Design review of the part built by this model. Coordinates are the model's own, in mm. Face numbers are marked on the shaded views. A direction names the side the tool comes from. Coordinates: 2 decimals unless noted, no trailing zeros. Order: outer loops, then holes, each group sorted by start corner. A loop starts at its lowest first (then second) coordinate and runs counter-clockwise, first axis right, second up. Notation, with made-up numbers: (31.25, 73) - (76.25, 73) arc R33 cw to (76.25, 108) - close; hole circle Ø6 at (-34.75, 49). An arc over 180 degrees is marked (long way). Write each question's results on one line, items separated by ' | '. Start each with the question number.
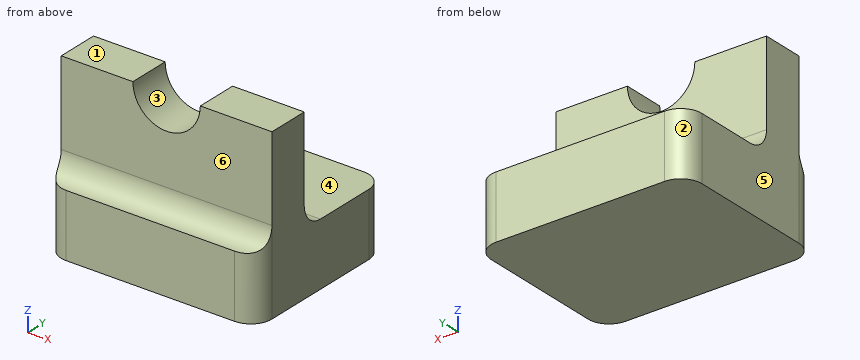
```python
from build123d import *

# Parameters (mm, degrees)
F0_W        = 50
F0_H        = 40
F1_DEPTH    = 15
F2_W        = 50
F2_H        = 10
F3_DEPTH    = 25
F5_DEPTH    = 25
F7_T1_DEPTH = 50
F7_T3_DEPTH = 40


# Not quite as in the source:
# - a fillet or chamfer that OpenCascade refuses, or shapes differently, is made with other operations: its cross-section is extruded or revolved along the edge and cut away or added
# - a feature of the source that left no trace in its solid (it failed there, or was rolled back) is left out


with BuildPart() as f1:
    # F0 (on Top) → F1 (new body)
    with BuildSketch(Plane.XY):
        with Locations((29.4554777443, -26.2415218353)):
            Rectangle(F0_W, F0_H)
    extrude(amount=F1_DEPTH)

    # F2 (on face) → F3 (join)
    with BuildSketch(Plane.XY.offset(15)):
        with Locations((29.4554777443, -36.2415218353)):
            Rectangle(F2_W, F2_H)
    extrude(amount=F3_DEPTH)

    # F4 (on face) → F5 (cut)
    with BuildSketch(Plane(origin=(0, -31.2415218353, 0), x_dir=(-1, 0, 0), z_dir=(0, 1, 0))):
        with BuildLine():
            ThreePointArc((-37.4554777443, 40), (-29.4554777443, 32), (-21.4554777443, 40))
            Line((-21.4554777443, 40), (-37.4554777443, 40))
        make_face()
    extrude(amount=-F5_DEPTH, mode=Mode.SUBTRACT)

    # F7: fillet of radius 5 on 6 edges, made by hand

    # F7_s2 → F7_t1 (join)
    with BuildSketch(Plane.YZ.offset(4.4554777443)):
        with BuildLine():
            ThreePointArc((-46.2415218353, 15), (-42.7059879294, 16.4644660941), (-41.2415218353, 20))
            Line((-41.2415218353, 20), (-41.2415218353, 15))
            Line((-41.2415218353, 15), (-46.2415218353, 15))
        make_face()
        with BuildLine():
            ThreePointArc((-26.2415218353, 15), (-29.7770557413, 16.4644660941), (-31.2415218353, 20))
            Line((-31.2415218353, 20), (-31.2415218353, 15))
            Line((-31.2415218353, 15), (-26.2415218353, 15))
        make_face()
    extrude(amount=F7_T1_DEPTH)

    # F7_s4 → F7_t3 (cut)
    with BuildSketch(Plane.XY.offset(-12.5)):
        with BuildLine():
            ThreePointArc((9.4554777443, -46.2415218353), (5.9199438384, -44.7770557413), (4.4554777443, -41.2415218353))
            Line((4.4554777443, -41.2415218353), (4.4554777443, -46.2415218353))
            Line((4.4554777443, -46.2415218353), (9.4554777443, -46.2415218353))
        make_face()
        with BuildLine():
            ThreePointArc((49.4554777443, -46.2415218353), (52.9910116503, -44.7770557413), (54.4554777443, -41.2415218353))
            Line((54.4554777443, -41.2415218353), (54.4554777443, -46.2415218353))
            Line((54.4554777443, -46.2415218353), (49.4554777443, -46.2415218353))
        make_face()
        with BuildLine():
            ThreePointArc((4.4554777443, -11.2415218353), (5.9199438384, -7.7059879294), (9.4554777443, -6.2415218353))
            Line((9.4554777443, -6.2415218353), (4.4554777443, -6.2415218353))
            Line((4.4554777443, -6.2415218353), (4.4554777443, -11.2415218353))
        make_face()
        with BuildLine():
            ThreePointArc((54.4554777443, -11.2415218353), (52.9910116503, -7.7059879294), (49.4554777443, -6.2415218353))
            Line((49.4554777443, -6.2415218353), (54.4554777443, -6.2415218353))
            Line((54.4554777443, -6.2415218353), (54.4554777443, -11.2415218353))
        make_face()
    extrude(amount=F7_T3_DEPTH, mode=Mode.SUBTRACT)


solid = f1.part
```
(1) Mouldability with a two-part tool opening along X and no side actions: class the marked faces 1, 2 and 3 as +X half, -X half, draft (parallel to the pull), parting line (faces both ways), or undercut.
(2) To check wall thickness, follow line 1 along Y through (x, z) = (20.5, 32.5); line 2 along Z through (x, y) = (33, -12.5); line 3 along Z through (x, y) = (13.5, -27.5). State the ranges of each line that lie inside material, in increasing order. Write a range as [from, to].
(3) Take a section at D-D (z = 22). State the section outline as (x, y) points, plus the area to 3 significant figures.
(4) Clearance check with flat-ended pins moving along their axes: pin 1 (6 mm diameter, centred on x = 28.5, y = -12, fed in from -Z); pin 2 (5 mm diameter, centred on x = 42, z = 32.5, fed in from -Y); pin 3 (22 mm diameter, centred on x = 21, y = -16.5, fed in from +Z); pin 4 (6 mm diameter, centred on x = 31, z = 27.5, fed in from +Y). State where each tip first meets the part, or that it passes through.
(5) Tool access review of the marked faces 4, 5 and 6: name each direction out of +Z, -Z, +X, -X, +Y, -Y from which nothing blocks a thin tool from reaching the whole face with its end or side.
(6) Take a section at A-A (x = 39). State the section outline as (y, z) points, plus the area to 3 significant figures.
(7) Take a section at C-C (y = -38). State the section outline as (x, z) points.
(8) Take a section at B-B (z = 36). State the section outline as (x, y) points.
Worked out:
1) face 1: draft | face 2: -X half | face 3: undercut
2) line 1: [-41.24, -31.24] | line 2: [0, 15] | line 3: [0, 15.16]
3) outline: (4.46, -41.24) - (54.46, -41.24) - (54.46, -31.24) - (4.46, -31.24) - close | area: 500 mm^2
4) pin 1: z = 0 | pin 2: y = -41.24 | pin 3: z = 15.16 | pin 4: y = -31.24
5) face 4: +Z, +X, -X, +Y | face 5: +Z, -Z, -X, +Y, -Y | face 6: +Z, +X, -X, -Y
6) outline: (-46.24, 0) - (-6.24, 0) - (-6.24, 15) - (-26.24, 15) arc R5 cw to (-31.24, 20) - (-31.24, 40) - (-41.24, 40) - (-41.24, 20) arc R5 cw to (-46.24, 15) - close | area: 861 mm^2
7) outline: (4.46, 0) - (54.46, 0) - (54.46, 40) - (37.46, 40) arc R8 cw to (21.46, 40) - (4.46, 40) - close
8) outline: (4.46, -41.24) - (22.53, -41.24) - (22.53, -31.24) - (4.46, -31.24) - close; (36.38, -41.24) - (54.46, -41.24) - (54.46, -31.24) - (36.38, -31.24) - close
